Read the model definition and answer for the solid it produces. Units are mm, in the model's axes. Coordinates: 2 decimals unless noted, no trailing zeros. Loops run counter-clockwise (first coordinate to the right, second up) from the corner with the lowest first, then second, coordinate; pieces in that order, holes last.
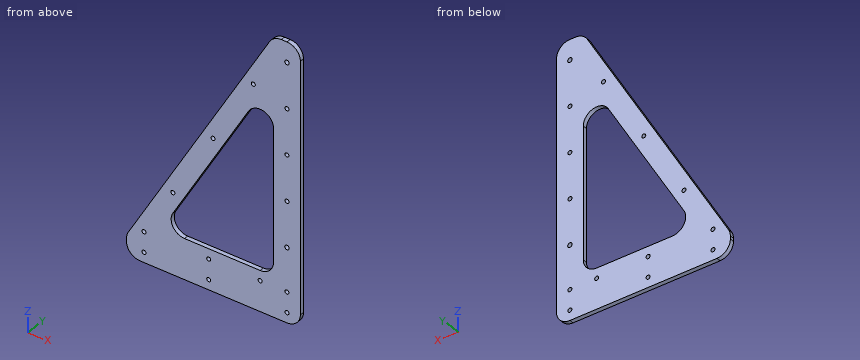
from build123d import *

# Parameters (mm, degrees)
SKETCH1_R           = 1.5
SKETCH1_R_2         = 1.65
BOSS_EXTRUDE1_DEPTH = 3.175
SKETCH2_W           = 129.696551146
SKETCH2_H           = 15
SKETCH2_R           = 1.5
BOSS_EXTRUDE2_DEPTH = 3.175
FILLET1_R           = 10


with BuildPart() as part:
    # Sketch1 → Boss-Extrude1 (new body)
    with BuildSketch(Plane(origin=(0, 0, 0), x_dir=(1, 0, 0), z_dir=(0, 1, 0))):
        Polygon((-20, -190), (0, -190), (0, 0), (-129.696551146, 0), align=None)
        with Locations(Location((-65.10548978, -96.875, 0), (0, 0, 270))):
            Circle(SKETCH1_R, mode=Mode.SUBTRACT)
        with Locations(Location((-10, -175, 0), (0, 0, 270))):
            Circle(SKETCH1_R_2, mode=Mode.SUBTRACT)
        with Locations(Location((-35.10548978, -148.836524227, 0), (0, 0, 270))):
            Circle(SKETCH1_R, mode=Mode.SUBTRACT)
        with BuildLine():
            ThreePointArc((-10, -139.75), (-8.5, -141.25), (-10, -142.75))
            ThreePointArc((-10, -142.75), (-11.5, -141.25), (-10, -139.75))
        make_face(mode=Mode.SUBTRACT)
        with BuildLine():
            ThreePointArc((-10, -106), (-8.5, -107.5), (-10, -109))
            ThreePointArc((-10, -109), (-11.5, -107.5), (-10, -106))
        make_face(mode=Mode.SUBTRACT)
        with Locations(Location((-95.10548978, -44.913475773, 0), (0, 0, 270))):
            Circle(SKETCH1_R, mode=Mode.SUBTRACT)
        with Locations(Location((-116.706170089, -7.5, 0), (0, 0, 270))):
            Circle(SKETCH1_R, mode=Mode.SUBTRACT)
        with Locations(Location((-68.353085045, -7.5, 0), (0, 0, 270))):
            Circle(SKETCH1_R, mode=Mode.SUBTRACT)
        Polygon((-20, -15), (-20, -160), (-103.715789032, -15), align=None, mode=Mode.SUBTRACT)
        with BuildLine():
            ThreePointArc((-10, -72.25), (-8.5, -73.75), (-10, -75.25))
            ThreePointArc((-10, -75.25), (-11.5, -73.75), (-10, -72.25))
        make_face(mode=Mode.SUBTRACT)
        with Locations(Location((-10, -40, 0), (0, 0, 270))):
            Circle(SKETCH1_R_2, mode=Mode.SUBTRACT)
        with Locations(Location((-30, -7.5, 0), (0, 0, 270))):
            Circle(SKETCH1_R, mode=Mode.SUBTRACT)
        with Locations(Location((-10, -7.5, 0), (0, 0, 270))):
            Circle(SKETCH1_R, mode=Mode.SUBTRACT)
    extrude(amount=BOSS_EXTRUDE1_DEPTH)

    # Sketch2 → Boss-Extrude2 (add)
    with BuildSketch(Plane.XZ):
        with Locations((-64.848275573, -7.5)):
            Rectangle(SKETCH2_W, SKETCH2_H)
        with Locations(Location((-116.706170089, -7.5, 0), (0, 0, 270))):
            Circle(SKETCH2_R, mode=Mode.SUBTRACT)
        with Locations(Location((-68.353085045, -7.5, 0), (0, 0, 270))):
            Circle(SKETCH2_R, mode=Mode.SUBTRACT)
        with Locations(Location((-10, -7.5, 0), (0, 0, 270))):
            Circle(SKETCH2_R, mode=Mode.SUBTRACT)
    extrude(amount=-BOSS_EXTRUDE2_DEPTH)

    # Fillet1
    fillet1_edges = [part.edges().sort_by_distance(p)[0] for p in [
        (0, 1.5875, 190),
        (-20, 1.5875, 190),
        (-129.696551146, 1.5875, 0),
        (-103.715789032, 1.5875, 15),
        (-20, 1.5875, 160),
        (-20, 1.5875, 15),
        (0, 1.5875, -15),
        (-129.696551146, 1.5875, -15),
    ]]
    fillet(fillet1_edges, radius=FILLET1_R)


solid = part.part
Item 1: A cutting plane is placed at C-C on z = 11. Determine the outline of the cut face in (x, y) (3 decimals).
Numbers:
outline: (-123.346, 0) - (0, 0) - (0, 3.175) - (-123.346, 3.175) - close
Item 2: A cutting plane is placed at A-A on z = 104. Determine the outline of the cut face in (x, y) (3 decimals).
Numbers:
outline: (-69.652, 0) - (-52.332, 0) - (-52.332, 3.175) - (-69.652, 3.175) - close; (-20, 0) - (0, 0) - (0, 3.175) - (-20, 3.175) - close
Item 3: A cutting plane is placed at D-D on z = 160. Determine the outline of the cut face in (x, y) (1 decimal), then the cut area to 3 significant figures.
Numbers:
outline: (-37.3, 0) - (0, 0) - (0, 3.2) - (-37.3, 3.2) - close
area: 118 mm2
Item 4: Find the intervals of material crossed by line 1 along X through (y, z) = (2.55, 7.5); line 2 along X through (y, z) = (0.7, 106.5); line 3 along X through (y, z) = (3, 73), in increasing order.
Numbers:
line 1: x = -125.37 to -118.21, -115.21 to -69.85, -66.85 to -31.5, -28.5 to -11.5, -8.5 to 0
line 2: x = -68.21 to -50.89, -20 to -11.12, -8.88 to 0
line 3: x = -87.55 to -70.23, -20 to -11.3, -8.7 to 0
Item 5: A cutting plane is placed at B-B on y = 1.25. Give the number of separate pieces and of enclosed holes in the cut face, then the cut area to 3 significant figures.
Numbers:
separate pieces: 1
enclosed holes: 16
area: 10,300 mm2
